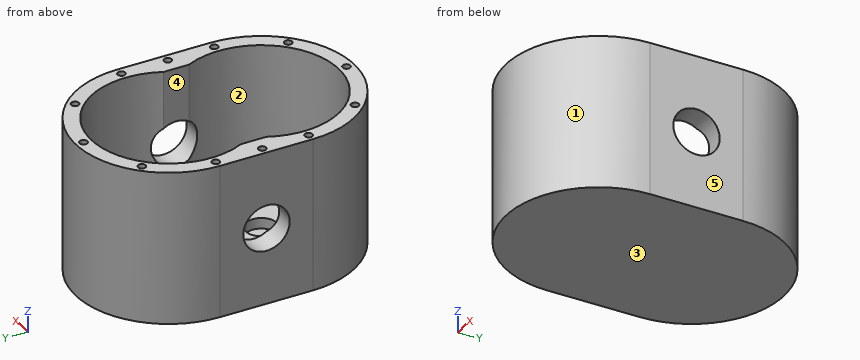
from build123d import *

# Parameters (mm, degrees)
OUTER_HOUSING_EXTRUDE_DEPTH            = 50
INNER_HOUSING_CUT_DEPTH                = 90
SKETCH3_R                              = 10
SHAFT_BEARING_INSERT_HOLE_DEPTH        = 7
HIGH_PRESSURE_OUTLET_HOLE_REACH        = 122
SKETCH4_R                              = 15
LOW_PRESSURE_INLET_HOLE_REACH          = 122
SKETCH5_R                              = 15
HOUSING_COVER_TOP_FASTENER_HOLES_COUNT = 8
M6X1_0_TAPPED_HOLE2_D                  = 5
M6X1_0_TAPPED_HOLE2_DEPTH              = 17
M6X1_0_TAPPED_HOLE2_TIP                = 1.502151548


with BuildPart() as part:
    # Sketch1 → Outer Housing Extrude (new body, symmetric)
    with BuildSketch(Plane.XY):
        with BuildLine():
            Line((-60, 30), (-60, -30))
            ThreePointArc((-60, -30), (0, -90), (60, -30))
            Line((60, -30), (60, 30))
            ThreePointArc((60, 30), (0, 90), (-60, 30))
        make_face()
    extrude(amount=OUTER_HOUSING_EXTRUDE_DEPTH, both=True)

    # Sketch2 → Inner Housing Cut (cut)
    with BuildSketch(Plane.XY.offset(50)):
        with BuildLine():
            Line((-45, 8.205505282), (-45, -8.205505282))
            ThreePointArc((-45, -8.205505282), (0, -80), (45, -8.205505282))
            Line((45, -8.205505282), (45, 8.205505282))
            ThreePointArc((45, 8.205505282), (0, 80), (-45, 8.205505282))
        make_face()
    extrude(amount=-INNER_HOUSING_CUT_DEPTH, mode=Mode.SUBTRACT)

    # Sketch3 → Shaft Bearing Insert Hole (cut)
    with BuildSketch(Plane.XY.offset(-40)):
        with Locations((0, 30)):
            Circle(SKETCH3_R)
        with Locations((0, -30)):
            Circle(SKETCH3_R)
    extrude(amount=-SHAFT_BEARING_INSERT_HOLE_DEPTH, mode=Mode.SUBTRACT)

    # Sketch4 → High Pressure Outlet Hole (cut, up to next)
    with BuildSketch(Plane.ZY.offset(60), mode=Mode.PRIVATE) as high_pressure_outlet_hole_sk1:
        Circle(SKETCH4_R)
    high_pressure_outlet_hole_tool1 = extrude(high_pressure_outlet_hole_sk1.sketch, amount=-HIGH_PRESSURE_OUTLET_HOLE_REACH, mode=Mode.PRIVATE) & part.part
    add(high_pressure_outlet_hole_tool1.solids().sort_by_distance((-60, 0, 0))[0], mode=Mode.SUBTRACT)

    # Sketch5 → Low Pressure Inlet Hole (cut, up to next)
    with BuildSketch(Plane(origin=(60, 0, 0), x_dir=(0, 0, -1), z_dir=(1, 0, 0)), mode=Mode.PRIVATE) as low_pressure_inlet_hole_sk1:
        Circle(SKETCH5_R)
    low_pressure_inlet_hole_tool1 = extrude(low_pressure_inlet_hole_sk1.sketch, amount=-LOW_PRESSURE_INLET_HOLE_REACH, mode=Mode.PRIVATE) & part.part
    add(low_pressure_inlet_hole_tool1.solids().sort_by_distance((60, 0, 0))[0], mode=Mode.SUBTRACT)

    # Sketch7 → M6x1.0 Tapped Hole1 (revolve, cut)
    with BuildSketch(Plane(origin=(0, 85, 50), x_dir=(0, -1, 0), z_dir=(1, 0, 0))):
        Polygon((0, 0), (0, 18.502151548), (2.5, 17), (2.5, 0), align=None)
    m6x1_0_tapped_hole1 = revolve(axis=Axis((0, 85, 56.35), (0, 0, -1)), mode=Mode.SUBTRACT)

    # Housing Cover Top Fastener Holes: M6x1.0 Tapped Hole1 ×8 about axis, 3 skipped
    housing_cover_top_fastener_holes_axis = Axis((0, 30, 0), (0, 0, 1))
    add([m6x1_0_tapped_hole1.rotate(housing_cover_top_fastener_holes_axis, i * 360 / HOUSING_COVER_TOP_FASTENER_HOLES_COUNT) for i in range(1, HOUSING_COVER_TOP_FASTENER_HOLES_COUNT) if i not in (3, 4, 5)], mode=Mode.SUBTRACT)

    # Housing Cover Bottom Fastener Holes: M6x1.0 Tapped Hole1 across plane
    add(m6x1_0_tapped_hole1.mirror(Plane.ZX), mode=Mode.SUBTRACT)

    # Housing Cover Bottom Fastener Holes copy → Housing Cover Bottom Fastener Holes  2 (revolve, cut)
    with BuildSketch(Plane(origin=(-38.890872965, -68.890872965, 50), x_dir=(0.707106781, 0.707106781, 0), z_dir=(0.707106781, -0.707106781, 0))):
        Polygon((0, 0), (0, -18.502151548), (2.5, -17), (2.5, 0), align=None)
    revolve(axis=Axis((-38.890872965, -68.890872965, 56.35), (0, 0, 1)), mode=Mode.SUBTRACT)

    # Housing Cover Bottom Fastener Holes  3 → Housing Cover Bottom Fastener Holes  4 (revolve, cut)
    with BuildSketch(Plane(origin=(-55, -30, 50), x_dir=(1, 0, 0), z_dir=(0, -1, 0))):
        Polygon((0, 0), (0, -18.502151548), (2.5, -17), (2.5, 0), align=None)
    revolve(axis=Axis((-55, -30, 56.35), (0, 0, 1)), mode=Mode.SUBTRACT)

    # Housing Cover Bottom Fastener Holes  5 → Housing Cover Bottom Fastener Holes  6 (revolve, cut)
    with BuildSketch(Plane(origin=(55, -30, 50), x_dir=(-1, 0, 0), z_dir=(0, 1, 0))):
        Polygon((0, 0), (0, -18.502151548), (2.5, -17), (2.5, 0), align=None)
    revolve(axis=Axis((55, -30, 56.35), (0, 0, 1)), mode=Mode.SUBTRACT)

    # Housing Cover Bottom Fastener Holes  7 → Housing Cover Bottom Fastener Holes  8 (revolve, cut)
    with BuildSketch(Plane(origin=(38.890872965, -68.890872965, 50), x_dir=(-0.707106781, 0.707106781, 0), z_dir=(0.707106781, 0.707106781, 0))):
        Polygon((0, 0), (0, -18.502151548), (2.5, -17), (2.5, 0), align=None)
    revolve(axis=Axis((38.890872965, -68.890872965, 56.35), (0, 0, 1)), mode=Mode.SUBTRACT)

    # M6x1.0 Tapped Hole2
    with Locations(Plane.XY.offset(50)):
        with Locations((-55, 0), (55, 0)):
            Hole(M6X1_0_TAPPED_HOLE2_D / 2, depth=M6X1_0_TAPPED_HOLE2_DEPTH)
            with Locations((0, 0, -(M6X1_0_TAPPED_HOLE2_DEPTH + M6X1_0_TAPPED_HOLE2_TIP / 2))):  # 118° drill point
                Cone(0, M6X1_0_TAPPED_HOLE2_D / 2, M6X1_0_TAPPED_HOLE2_TIP, mode=Mode.SUBTRACT)


solid = part.part
The listing builds one solid part. Answer for the finished solid, in the listing's coordinates (mm). Face numbers are marked on the shaded views. A direction names the side the tool comes from. Round coordinates to 2 decimals unless told otherwise and drop trailing zeros. Write each loop counter-clockwise with the first axis right and the second up, starting at its lowest first coordinate (ties: lowest second). Pieces come first, ordered by that corner, then holes. Notation, with made-up numbers: M 34.5,85.5 L 82.5,85.5 A15 ccw 82.5,95.5 Z; hole C 13,72 d2. An arc over 180 degrees is marked long. Write each question's results on one line, items separated by ' | '. Start each with the question number.
Item 1: Find section C-C on x = -27. Write down the section's boundary in (y, z).
Item 2: Straight lines are drawn through the part: probe 1 along Y at (x, z) = (0, 43); probe 2 along Y at (x, z) = (-55, 45); probe 3 along Y at (x, z) = (0, -19). For each, find the intervals that lie inside material, in ascending order.
Item 3: Find section D-D on y = 58. Write down the section's boundary in (x, z), and give its area (3 significant figures).
Item 4: Given pin 1 Ø8 at (x, y) = (11, -57.5) entering from +Z; pin 2 Ø10 at (y, z) = (-40, -38) entering from +X; pin 3 Ø4 at (y, z) = (-44.5, -13) entering from +X, each flat-ended and moving along its own axis, determine where each tip first touches the part or whether it passes through.
Item 5: Find section B-B on z = -3.5. Write down the section's boundary in (x, y).
Item 6: Find section A-A on z = 21. Write down the section's boundary in (x, y).
Item 7: The mould has two halves that part along Y. Classify the marked faces 1, 2 and 3: +Y half, -Y half, draft (parallel to the pull), parting line (faces both ways), or undercut.
Item 8: Which of the six approach directions +Z, -Z, +X, -X, +Y, -Y give full straight-line access (tool end or side, diameter ignored) to the marked faces 4 and 5?
Answer block:
1) outline: M -83.58,-50 L 83.58,-50 L 83.58,50 L 72.08,50 L 72.08,-40 L -72.08,-40 L -72.08,50 L -83.58,50 Z
2) probe 1: y = -90 to -87.5, -82.5 to -80, 80 to 82.5, 87.5 to 90 | probe 2: y = -53.98 to -32.5, -27.5 to -2.5, 2.5 to 27.5, 32.5 to 53.98 | probe 3: y = -90 to -80, 80 to 90
3) outline: M -53.07,-50 L 53.07,-50 L 53.07,50 L 41.42,50 L 41.42,-40 L -41.42,-40 L -41.42,50 L -53.07,50 Z | area: 3,160 mm²
4) pin 1: stops at z = -40 | pin 2: stops at x = 59.79 | pin 3: stops at x = 58.68
5) outline: M -60,-30 A60 ccw 60,-30 L 60,-14.59 L 47.56,-14.59 A50 cw long -47.56,-14.59 L -60,-14.59 Z; M -60,14.59 L -47.56,14.59 A50 cw long 47.56,14.59 L 60,14.59 L 60,30 A60 ccw -60,30 Z
6) outline: M -60,-30 A60 ccw 60,-30 L 60,30 A60 ccw -60,30 Z; hole M -45,-8.21 A50 ccw long 45,-8.21 L 45,8.21 A50 ccw long -45,8.21 Z
7) face 1: -Y half | face 2: undercut | face 3: draft
8) face 4: +Z | face 5: +Z, -Z, +X, +Y, -Y
